For this review, take the finished solid that the model builds, in its own axes (mm). Face numbers are marked on the shaded views. A direction names the side the tool comes from. Give positions to 0.01 mm unless a question says otherwise; leave off trailing zeros. Order: outer loops, then holes, each group sorted by start corner. A loop starts at its lowest first (then second) coordinate and runs counter-clockwise, first axis right, second up.
Item 1: Machinability: for the marked faces 5 and 6, which of the approach directions +Z, -Z, +X, -X, +Y, -Y give a long, thin tool a straight path to every point of the face, cutting with its end or side? Answer none if there is none.
Item 2: For P1, Ø3, axis at y = 28, z = -13, coming from the +X side; P2, Ø5, axis at x = -108, z = -8, coming from the -Y side; P3, Ø5, axis at y = 15.5, z = -7.5, coming from the +X side, all flat-tipped, find the tip position at first contact; note any pin that passes through.
Item 3: Consider section A-A (z = 0). Give the boundary of the cut face in (x, y).
Item 4: Consider section D-D (x = -106.5). Give the boundary of the cut face in (y, z), plus the area to 3 significant figures.
Item 5: The part is to be moulded in two halves that separate along Z. For the marked faces 1, 2, 3 and 4, say which applies: released by +Z, released by -Z, zero draft, split by the parting line, or undercut.
Item 6: For probe 1 along X at (y, z) = (38, 0); probe 2 along Y at (x, z) = (-117, 7); probe 3 along Z at (x, y) = (-112.5, 19), list the stretches that pass through material, from the lowest coordinate up.
Item 7: Consider section C-C (y = 31). Give the boundary of the cut face in (x, z).
Item 8: Consider section B-B (x = -96). Give the boundary of the cut face in (y, z).
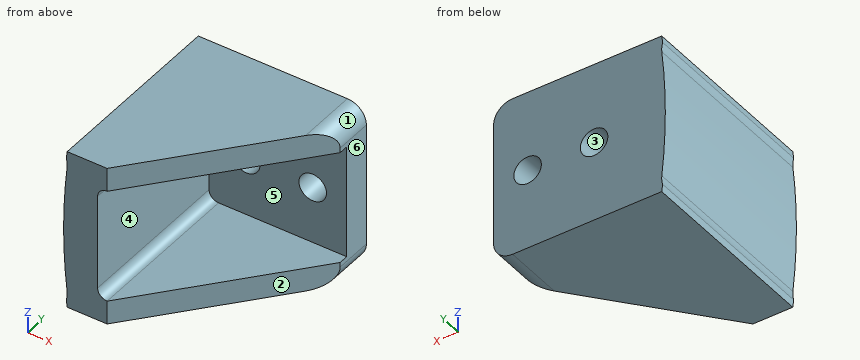
```python
from build123d import *

# Parameters (mm, degrees)
BOSS_EXTRUDE1_DEPTH = 40
CUT_EXTRUDE1_REACH  = 137.577
SKETCH3_W           = 29
SKETCH3_H           = 24
CUT_EXTRUDE2_DEPTH  = 34
SKETCH6_R           = 2.9
CUT_EXTRUDE3_DEPTH  = 31
FILLET2_R           = 4
BOSS_EXTRUDE3_START = -40
BOSS_EXTRUDE3_DEPTH = 40
FILLET4_R           = 5
FILLET5_R           = 2


with BuildPart() as part:
    # Sketch1 → Boss-Extrude1 (new body)
    with BuildSketch(Plane(origin=(0, 0, 0), x_dir=(1, 0, 0), z_dir=(0, 1, 0))):
        with BuildLine():
            Line((-123.838604643, 17), (-88.838604643, 17))
            Line((-88.838604643, 17), (-88.838604643, -17))
            Line((-88.838604643, -17), (-123.838604643, -17))
            ThreePointArc((-123.838604643, -17), (-125, 0), (-123.838604643, 17))
        make_face()
    extrude(amount=BOSS_EXTRUDE1_DEPTH)

    # Sketch2 → Cut-Extrude1 (cut, up to next)
    with BuildSketch(Plane.XY.offset(17), mode=Mode.PRIVATE) as cut_extrude1_sk1:
        Polygon((-88.838604643, 0), (-88.838604643, 32), (-115.838604643, 0), align=None)
    cut_extrude1_tool1 = extrude(cut_extrude1_sk1.sketch, amount=-CUT_EXTRUDE1_REACH, mode=Mode.PRIVATE) & part.part
    add(cut_extrude1_tool1.solids().sort_by_distance((-97.838605, 10.666667, 17))[0], mode=Mode.SUBTRACT)

    # Sketch3 → Cut-Extrude2 (cut)
    with BuildSketch(Plane.XZ):
        with Locations((-103.338604643, 0)):
            Rectangle(SKETCH3_W, SKETCH3_H)
    extrude(amount=-CUT_EXTRUDE2_DEPTH, mode=Mode.SUBTRACT)

    # Sketch6 → Cut-Extrude3 (cut)
    with BuildSketch(Plane(origin=(0, 40, 0), x_dir=(1, 0, 0), z_dir=(0, 1, 0))):
        with Locations(Location((-110, 0, 0), (0, 0, 270))):
            Circle(SKETCH6_R)
        with Locations(Location((-96, 0, 0), (0, 0, 270))):
            Circle(SKETCH6_R)
    extrude(amount=-CUT_EXTRUDE3_DEPTH, mode=Mode.SUBTRACT)

    # Fillet2
    fillet2_edges = [part.edges().sort_by_distance(p)[0] for p in [
        (-88.838604643, 36, -17),
        (-88.838604643, 36, 17),
    ]]
    fillet(fillet2_edges, radius=FILLET2_R)

    # Sketch8 → Boss-Extrude3 (add)
    with BuildSketch(Plane(origin=(0, 40, 0), x_dir=(1, 0, 0), z_dir=(0, 1, 0)).offset(BOSS_EXTRUDE3_START)):
        with BuildLine():
            Line((-123.838604643, 17), (-124.242343829, 17))
            ThreePointArc((-124.242343829, 17), (-124.342622992, 16.250295609), (-124.438378324, 15.5))
            Line((-124.438378324, 15.5), (-124.03527724, 15.5))
            ThreePointArc((-124.03527724, 15.5), (-123.93921022, 16.250297537), (-123.838604643, 17))
        make_face()
        with BuildLine():
            Line((-124.438378324, -15.5), (-124.03527724, -15.5))
            ThreePointArc((-124.03527724, -15.5), (-123.93921022, -16.250297537), (-123.838604643, -17))
            Line((-123.838604643, -17), (-124.242343829, -17))
            ThreePointArc((-124.242343829, -17), (-124.342622992, -16.250295609), (-124.438378324, -15.5))
        make_face()
    extrude(amount=BOSS_EXTRUDE3_DEPTH)

    # Fillet4
    # the kernel refuses this fillet: 5 mm, written as the material it adds along each edge
    with BuildSketch(Plane(origin=(-124.03527724, 0, 15.5), x_dir=(-0.11618374288163974, 0, -0.9932277371731083), z_dir=(0, 1, 0))) as fillet4_piece_1:
        with BuildLine():
            CenterArc((2.007660221, 4.99984503), FILLET4_R, 246.910702944, 22.638192563)
            Line((0.046833793, 0.400371178), (0.007617264, 0.308381701))
            ThreePointArc((0.007617264, 0.308381701), (-0.075905877, 0.211803963), (-0.099322774, 0.011618374))
            Line((-0.099322774, 0.011618374), (0.000787318, -0.099996901))
            ThreePointArc((0.000787318, -0.099996901), (0.984147167, -0.096125757), (1.967507016, -0.099996901))
            Line((1.967507016, -0.099996901), (1.968294334, 0))
        make_face()
    extrude(amount=40)
    with BuildSketch(Plane(origin=(-124.03527724, 0, -15.5), x_dir=(-1, 0, 0), z_dir=(0, 1, 0))) as fillet4_piece_2:
        with BuildLine():
            CenterArc((5.199242245, 1.413163109), FILLET4_R, 173.779198266, 22.638192563)
            Line((0.228683803, 1.954964528), (0.129272634, 1.965800556))
            ThreePointArc((0.129272634, 1.965800556), (0.018867133, 0.988650514), (-0.099228222, 0.0124))
            Line((-0.099228222, 0.0124), (0, -0.1))
            ThreePointArc((0, -0.1), (0.201550542, -0.1), (0.307178261, -0.028263262))
            Line((0.307178261, -0.028263262), (0.403101084, 0))
        make_face()
    extrude(amount=40)

    # Fillet5
    fillet5_edges = [part.edges().sort_by_distance(p)[0] for p in [
        (-117.838604643, 17, 12),
        (-117.838604643, 17, -12),
    ]]
    fillet(fillet5_edges, radius=FILLET5_R)


solid = part.part
```
Resolved:
1. face 5: +X, -Y
1. face 6: +Z, -Z, +X, +Y, -Y
2. P1: stops at x = -90.95
2. P2: stops at y = 34
2. P3: stops at x = -117.84
3. outline: (-125, 0) - (-117.84, 0) - (-117.84, 34) - (-112.9, 34) - (-112.9, 40) - (-125, 40) - close; (-107.1, 34) - (-98.9, 34) - (-98.9, 40) - (-107.1, 40) - close; (-93.1, 34) - (-88.84, 34) - (-88.84, 40) - (-93.1, 40) - close
4. outline: (11.07, -17) - (40, -17) - (40, 17) - (11.07, 17) - (11.07, 12) - (34, 12) - (34, -12) - (11.07, -12) - close
4. area: 433 mm2
5. face 1: released by +Z
5. face 2: zero draft
5. face 3: undercut
5. face 4: undercut
6. probe 1: x = -125 to -112.9, -107.1 to -98.9, -93.1 to -88.84
6. probe 2: y = 34 to 40
6. probe 3: z = -17 to -12, 12 to 17
7. outline: (-124.44, -15.5) arc R125.4 ccw to (-124.24, -17) - (-92.84, -17) arc R4 ccw to (-89.68, -15.46) - (-89.68, -12) - (-115.84, -12) arc R2 cw to (-117.84, -10) - (-117.84, 10) arc R2 cw to (-115.84, 12) - (-89.68, 12) - (-89.68, 15.46) arc R4 ccw to (-92.84, 17) - (-124.24, 17) arc R125.4 ccw to (-124.44, 15.5) arc R5 cw to (-124.26, 13.55) arc R125 ccw to (-124.26, -13.55) arc R5 cw to start
8. outline: (23.51, -17) - (40, -17) - (40, -2.9) - (34, -2.9) - (34, -12) - (23.51, -12) - close; (23.51, 12) - (34, 12) - (34, 2.9) - (40, 2.9) - (40, 17) - (23.51, 17) - close
